Work out the finished part from the listing and answer in its coordinate system (mm). Face numbers are marked on the shaded views. Coordinates: 2 decimals unless noted, no trailing zeros. Order: outer loops, then holes, each group sorted by start corner. A loop starts at its lowest first (then second) coordinate and runs counter-clockwise, first axis right, second up. Notation, with made-up numbers: (42.25, 44.5) -> (74.25, 44.5) arc R29 ccw to (74.25, 72.5) -> close; hole circle Ø11 at (13.25, 51). An arc over 180 degrees is marked (long way). Use one line per item in the form item = value.
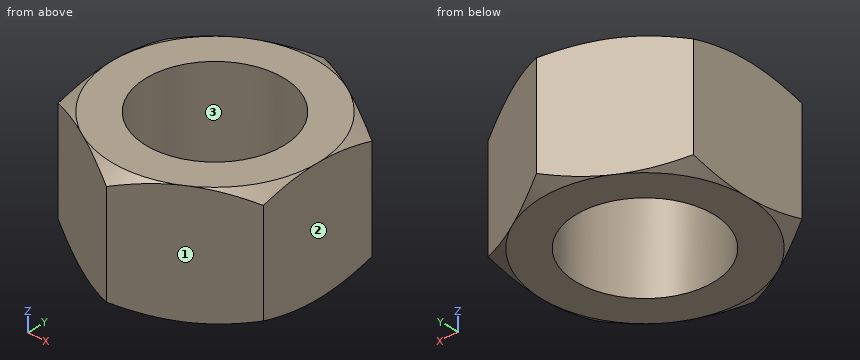
from build123d import *

# Parameters (mm, degrees)
SKETCH1_R               = 7.9375
EXTRUDE1_DEPTH          = 6.9453125
SKETCH7_OUTSIDE_W       = 121.588
SKETCH7_OUTSIDE_H       = 125.272
SKETCH7_OUTSIDE_R       = 11.90625
EXTRUDE2_DEPTH          = 25.4
EXTRUDE2_DRAFT          = -60
MIRROR1_COPY_1_SKETCH_W = 121.588
MIRROR1_COPY_1_SKETCH_H = 125.272
MIRROR1_COPY_1_SKETCH_R = 11.90625
MIRROR1_COPY_1_DEPTH    = 25.4
MIRROR1_COPY_1_DRAFT    = -60


with BuildPart() as part:
    # Sketch1 → Extrude1 (new, symmetric)
    with BuildSketch(Plane.XY):
        Polygon((-11.90625, 6.874076643), (-11.90625, -6.874076643), (0, -13.748153285), (11.90625, -6.874076643), (11.90625, 6.874076643), (0, 13.748153285), align=None)
        Circle(SKETCH1_R, mode=Mode.SUBTRACT)
    extrude(amount=EXTRUDE1_DEPTH, both=True)


with BuildPart() as extrude2_tool:
    # Sketch7 outside → Extrude2 (with draft: the straight prism first)
    with BuildSketch(Plane.XY.offset(6.9453125)):
        Rectangle(SKETCH7_OUTSIDE_W, SKETCH7_OUTSIDE_H)
        Circle(SKETCH7_OUTSIDE_R, mode=Mode.SUBTRACT)
    extrude(amount=-EXTRUDE2_DEPTH)
    # Extrude2: the draft: its side faces are tilted about the plane it starts from
    extrude2_sides = [extrude2_tool.faces().sort_by_distance(p)[0] for p in [
        (0, -62.636, -5.7546875),
        (60.794, 0, -5.7546875),
        (0, 62.636, -5.7546875),
        (-60.794, 0, -5.7546875),
        (-11.90625, 0, -5.7546875),
    ]]
    draft(extrude2_sides, Plane.XY.offset(6.9453125), EXTRUDE2_DRAFT)


with BuildPart() as part_1:
    add(part.part)

    # Extrude2: cut by extrude2_tool
    add(extrude2_tool.part, mode=Mode.SUBTRACT)


with BuildPart() as mirror1_copy_1_tool:
    # Mirror1 copy 1 sketch → Mirror1 copy 1 (with draft: the straight prism first)
    with BuildSketch(Plane(origin=(0, 0, -6.9453125), x_dir=(1, 0, 0), z_dir=(0, 0, -1))):
        Rectangle(MIRROR1_COPY_1_SKETCH_W, MIRROR1_COPY_1_SKETCH_H)
        Circle(MIRROR1_COPY_1_SKETCH_R, mode=Mode.SUBTRACT)
    extrude(amount=-MIRROR1_COPY_1_DEPTH)
    # Mirror1 copy 1: the draft: its side faces are tilted about the plane it starts from
    mirror1_copy_1_sides = [mirror1_copy_1_tool.faces().sort_by_distance(p)[0] for p in [
        (0, -62.636, 5.7546875),
        (60.794, 0, 5.7546875),
        (0, 62.636, 5.7546875),
        (-60.794, 0, 5.7546875),
        (-11.90625, 0, 5.7546875),
    ]]
    draft(mirror1_copy_1_sides, Plane(origin=(0, 0, -6.9453125), x_dir=(1, 0, 0), z_dir=(0, 0, -1)), MIRROR1_COPY_1_DRAFT)


with BuildPart() as part_2:
    add(part_1.part)

    # Mirror1 copy 1: cut by mirror1_copy_1_tool
    add(mirror1_copy_1_tool.part, mode=Mode.SUBTRACT)


solid = part_2.part
(1) Section A-A on z = -3 is taken. Write down the section's boundary in (x, y) (1 decimal), plus the area to 3 significant figures.
Data:
outline = (-11.9, -6.9) -> (0, -13.7) -> (11.9, -6.9) -> (11.9, 6.9) -> (0, 13.7) -> (-11.9, 6.9) -> close; hole circle Ø15.9 at (0, 0)
area = 293 mm²
(2) Section B-B on z = 6.25 is taken. Write down the section's boundary in (x, y) (1 decimal).
Data:
outline = (-11.9, -5.5) arc R13.1 ccw to (-10.7, -7.6) -> (-1.2, -13.1) arc R13.1 ccw to (1.2, -13.1) -> (10.7, -7.6) arc R13.1 ccw to (11.9, -5.5) -> (11.9, 5.5) arc R13.1 ccw to (10.7, 7.6) -> (1.2, 13.1) arc R13.1 ccw to (-1.2, 13.1) -> (-10.7, 7.6) arc R13.1 ccw to (-11.9, 5.5) -> close; hole circle Ø15.9 at (0, 0)
(3) Straight lines are drawn through the part: line 1 along X through (y, z) = (-0.25, 4.5); line 2 along Z through (x, y) = (2, -11.75); line 3 along Y through (x, z) = (2, 3.5). For each, find the intervals that lie inside material, in ascending order.
Data:
line_1 = -11.91 to -7.93, 7.93 to 11.91
line_2 = -6.94 to 6.94
line_3 = -12.59 to -7.68, 7.68 to 12.59
(4) Each of these flat-tipped pins is pushed along its axis until it touches: P1, Ø12, axis at x = -0.5, y = -7.5, coming from the -Z side; P2, Ø1, axis at x = 2.5, z = 0, coming from the -Y side. Where does it stop, or does it pass through?
Data:
P1 = -6.95
P2 = -12.59
(5) The mould has two halves that part along Y. Classify the marked faces 1, 2 and 3: released by +Y, released by -Y, zero draft, split by the parting line, or undercut.
Data:
face_1 = released by -Y
face_2 = zero draft
face_3 = undercut
